Build history of the part. All positions in model axes, mm. A direction names the side the tool comes from. Coordinates: 2 decimals unless noted, no trailing zeros. Order: outer loops, then holes, each group sorted by start corner. A loop starts at its lowest first (then second) coordinate and runs counter-clockwise, first axis right, second up. Notation, with made-up numbers: (72.25, 76.5) - (122.25, 76.5) arc R37 ccw to (122.25, 114.5) - close; hole circle Ø10 at (25, -39.75). An arc over 180 degrees is marked (long way). Write each question's results on one line, items separated by ' | '.
from build123d import *


with BuildPart() as part:
    # Sketch1 → Revolve1 (revolve)
    with BuildSketch(Plane.XZ, mode=Mode.PRIVATE) as revolve1_sk:
        with BuildLine():
            Line((7.5, 14.5), (0, 14.5))
            Line((0, 14.5), (0, 0))
            Line((0, 0), (45, 0))
            ThreePointArc((45, 0), (48.535533906, 1.464466094), (50, 5))
            Line((50, 5), (50, 38))
            ThreePointArc((50, 38), (48.535533906, 41.535533906), (45, 43))
            Line((45, 43), (37, 43))
            Line((37, 43), (37, 20.5))
            Line((37, 20.5), (7.5, 20.5))
            Line((7.5, 20.5), (7.5, 14.5))
        make_face()
    revolve(revolve1_sk.sketch.rotate(Axis((0, 0, 43), (0, 0, -1)), 180), axis=Axis((0, 0, 43), (0, 0, -1)))


solid = part.part
1. Band-saw the part on A-A on z = 29.5. Give the cut face in (x, y), then the cut area to 3 significant figures.
Solved:
outline: circle Ø100 at (0, 0); hole circle Ø74 at (0, 0) | area: 3,550 mm2
2. Band-saw the part on B-B on y = 0. Give the cut face in (x, z), then the cut area to 3 significant figures.
Solved:
outline: (-50, 5) arc R5 ccw to (-45, 0) - (45, 0) arc R5 ccw to (50, 5) - (50, 38) arc R5 ccw to (45, 43) - (37, 43) - (37, 20.5) - (7.5, 20.5) - (7.5, 14.5) - (-7.5, 14.5) - (-7.5, 20.5) - (-37, 20.5) - (-37, 43) - (-45, 43) arc R5 ccw to (-50, 38) - close | area: 2,520 mm2
3. Band-saw the part on D-D on z = 16. Give the cut face in (x, y), then the cut area to 3 significant figures.
Solved:
outline: circle Ø100 at (0, 0); hole circle Ø15 at (0, 0) | area: 7,680 mm2
4. Two-plate mould, pull along X, no slides. Class faces 3 (the face through (-47.69, 15.02, 21.73)), 4 (the face through (10, -36, 43)), 5 (the face through (-4.032, 6.324, 17.458)): +X half, -X half, draft (parallel to the pull), parting line (faces both ways), or undercut.
Solved:
face 3: parting line | face 4: draft | face 5: undercut
5. Drop flat-ended pins along their axis: pin 1 Ø1 at (x, z) = (-35, 10.5) entering from +Y; pin 2 Ø1.5 at (y, z) = (6.5, 25) entering from -X; pin 3 Ø8 at (y, z) = (-7, 28.5) entering from -X. Give the stop position or say it passes through.
Solved:
pin 1: stops at y = 36.19 | pin 2: stops at x = -49.67 | pin 3: stops at x = -49.91
6. Tool access for faces 1 (the face through (-1, 1, 0)), 2 (the face through (-8, 1, 20.5)): list every direction of +Z, -Z, +X, -X, +Y, -Y with a clear straight run to the whole face (end or side of a thin tool).
Solved:
face 1: -Z, +X, -X, +Y, -Y | face 2: +Z
7. Probe line 1 (Y direction, x = 0, z = 32); line 2 (Z direction, x = 26, y = -5); line 3 (Y direction, x = 33, z = 35). List the from-to ranges inside material, lowest first.
Solved:
line 1: y = -50 to -37, 37 to 50 | line 2: z = 0 to 20.5 | line 3: y = -37.56 to -16.73, 16.73 to 37.56
